Input: part model. Units: mm. Frame: model coordinates. A direction names the side the tool comes from. Coordinates: 2 decimals unless noted, no trailing zeros. Write each loop counter-clockwise with the first axis right and the second up, starting at its lowest first coordinate (ties: lowest second). Pieces come first, ordered by that corner, then holes. Notation, with made-up numbers: M 29,-12 L 72,-12 A11 cw 72,4 Z; hole C 79,-19.5 d8. An arc over 180 degrees is marked long. Write each question's results on one line, items separated by ' | '. Start each with the question number.
1. Section query D-D, the plane x = -34. Output: boundary loops of the cut face in (y, z).
2. Section query C-C, the plane x = -98. Output: boundary loops of the cut face in (y, z), and give its area (3 significant figures).
3. Pull-direction query (X, two-part tool) for faces 1 (the flat face through (108, -23, 25.251)), 2 (the flat face through (152.4, -18, -1)), 3 (the flat face through (-2, -18, -44.45)); classes: +X half, -X half, draft (parallel to the pull), parting line (faces both ways), or undercut.
4. Ray query, probe 1 along X at (y, z) = (-23.5, 31.5); probe 2 along Z at (x, y) = (103, -20); probe 3 along X at (y, z) = (-21.5, -2). Return the intervals inside material, ascending.
5. Section query B-B, the plane z = -16.5. Output: boundary loops of the cut face in (x, y), and give its area (3 significant figures).
6. Set-up query: faces 4 (the flat face through (74.999, -23, 35)), 5 (the flat face through (141.857, -23, 0)), 6 (the flat face through (-1, -35.56, -29)). Return all of +Z, -Z, +X, -X, +Y, -Y with unobstructed straight access to the full face (end or side cutting, diameter ignored); none if empty.
7. Section query A-A, the plane y = -28. Output: boundary loops of the cut face in (x, z).
```python
from build123d import *

# Parameters (mm, degrees)
F0_W     = 304.8
F0_H     = 88.9
F1_DEPTH = 35.56
F3_DEPTH = 25.4
F4_DEPTH = 25.4
F2_W     = 66.8579302463
F2_H     = 50.5015006546
F2_W_2   = 66.8579153451
F5_DEPTH = 25.4


# Not quite as in the source:
# - a feature names something its author has since deleted; it is built from what else it names


with BuildPart() as f1:
    # F0 (on Front) → F1 (new body)
    with BuildSketch(Plane.XZ):
        Rectangle(F0_W, F0_H)
    extrude(amount=F1_DEPTH)

    # F2 (on face) → F3 (cut)
    with BuildSketch(Plane.XZ.offset(35.56)):
        Polygon((-33.3375, 19.1518365622), (-33.3375, 44.45), (-74.9989692254, 44.45), (-74.9989692254, 25.2507503273), (-74.9989692254, -25.2507503273), (74.9989692254, -25.2507503273), (74.9989692254, 25.2507503273), (74.9989692254, 44.45), (33.3375, 44.45), (33.3375, 19.1518365622), align=None)
    extrude(amount=-F3_DEPTH, mode=Mode.SUBTRACT)

    # F4 (cut): a face of the model
    f4_faces = [f1.faces().sort_by_distance(p)[0] for p in [
        (0, -35.56, 31.8009182811),
    ]]
    extrude(f4_faces, amount=-F4_DEPTH, mode=Mode.SUBTRACT)

    # F2 (on face) → F5 (cut)
    with BuildSketch(Plane.XZ.offset(35.56)):
        with Locations((-108.4279343486, 0)):
            Rectangle(F2_W, F2_H)
        with Locations((108.427926898, 0)):
            Rectangle(F2_W_2, F2_H)
    extrude(amount=-F5_DEPTH, mode=Mode.SUBTRACT)


solid = f1.part
```
Answer:
1) outline: M -35.56,-44.45 L 0,-44.45 L 0,44.45 L -10.16,44.45 L -10.16,-25.25 L -35.56,-25.25 Z
2) outline: M -35.56,-44.45 L 0,-44.45 L 0,44.45 L -35.56,44.45 L -35.56,25.25 L -10.16,25.25 L -10.16,-25.25 L -35.56,-25.25 Z | area: 1,880 mm^2
3) face 1: undercut | face 2: +X half | face 3: draft
4) probe 1: -152.4 to -75, 75 to 152.4 | probe 2: -44.45 to -25.25, 25.25 to 44.45 | probe 3: -152.4 to -141.86, 141.86 to 152.4
5) outline: M -152.4,-35.56 L -141.86,-35.56 L -141.86,-10.16 L 141.86,-10.16 L 141.86,-35.56 L 152.4,-35.56 L 152.4,0 L -152.4,0 Z | area: 3,630 mm^2
6) face 4: +Z, -Y | face 5: -Y | face 6: +Z, -Z, +X, -X, -Y
7) outline: M -152.4,-44.45 L 152.4,-44.45 L 152.4,44.45 L 75,44.45 L 75,25.25 L 141.86,25.25 L 141.86,-25.25 L -141.86,-25.25 L -141.86,25.25 L -75,25.25 L -75,44.45 L -152.4,44.45 Z
